Solid Edge part; units mm, degrees
sketch "Sketch1" plane through (0, 0, 0) normal (1, 0, 0) x (0, 1, 0)
  line L0 (0, 50) -> (0, 31)
  line L1 (0, 31) -> (-5, 31)
  line L2 (-5, 31) -> (-5, 26.5)
  line L3 (-5, 26.5) -> (0, 26.5)
  line L4 (0, 26.5) -> (0, 21)
  line L5 (0, 21) -> (4, 21)
  line L6 (4, 21) -> (4, 22.5)
  line L7 (4, 22.5) -> (11, 22.5)
  line L8 (11, 22.5) -> (11, 31)
  line L9 (11, 31) -> (8, 31)
  line L10 (8, 32.5) -> (8, 31)
  line L11 (8, 39) -> (8, 32.5)
  line L12 (8, 39) -> (8, 50)
  line L13 (8, 50) -> (0, 50)
revolve "RevolvedProtrusion1" add sketch "Sketch1" angle 360 about axis through (0, -22.1591, 0) along (0, 1, 0)
sketch "Sketch2" plane through (0, 8, 0) normal (0, 1, 0) x (-1, 0, 0)
  circle A0 centre (-28.2843, -28.2843) radius 4.25
  circle A1 centre (-28.2843, 28.2843) radius 4.25
  circle A2 centre (28.2843, 28.2843) radius 4.25
  circle A3 centre (28.2843, -28.2843) radius 4.25
extrude "Cutout1" cut sketch "Sketch2" against normal blind 16.0733
Check sheet for the modelled part. Datum: model origin and axes. Units: mm. A direction names the side the tool comes from. Coordinates: 2 decimals unless noted, no trailing zeros. Loops run counter-clockwise (first coordinate to the right, second up) from the corner with the lowest first, then second, coordinate; pieces in that order, holes last. Notation, with made-up numbers: (46.5, -35.75) -> (105.5, -35.75) arc R5 ccw to (105.5, -31.75) -> close; hole circle Ø3 at (10, 52). An arc over 180 degrees is marked (long way). Write item = value, one per line. Start each with the question number.
1. Material ranges on line 1 (Z direction, x = -27, y = 5); line 2 (X direction, y = 7.25, z = 0); line 3 (Y direction, x = 33.5, z = 16), recorded low to high.
2. Section check D-D on y = 9.5. Record the cut outline in (x, z), then the cut area to 3 significant figures.
3. Section check B-B on x = 0. Record the cut outline in (y, z), then the cut area to 3 significant figures.
4. Section check A-A on z = 0. Record the cut outline in (x, y).
5. Depth check by flat-ended pin: P1, Ø5, axis at x = 28.28, z = 28.28, coming from the -Y side; P2, Ø16, axis at x = -12, z = 5.5, coming from the -Y side; P3, Ø8, axis at x = -35, y = 0.5, coming from the -Z side; P4, Ø2, axis at y = -3, z = 6.5, coming from the -X side. Enter the tip coordinate at first touch or a pass-through.
6. Tool access check on faces 4 (the flat face through (14, -5, 23)), 5 (the cylindrical face through (-30.736, -2.535, -4.036)), 6 (the flat face through (-22, 8, -23)). Record the directions out of +Z, -Z, +X, -X, +Y, -Y that give a thin tool (end or side, any length) a straight path to the whole face; none if there is none.
7. Section check C-C on y = -2.75. Record the cut outline in (x, z), then the cut area to 3 significant figures.
8. Draft check along Z on faces 1 (the cylindrical face through (-30.736, 9.479, -4.036)), 2 (the flat face through (7, 4, 20)), 3 (the flat face through (-22, 0, -23)). Enter one of: released by +Z, released by -Z, zero draft, split by the parting line, or undercut.
Responses:
q1.line_1 = -42.08 to -32.34, -24.23 to 24.23, 32.34 to 42.08
q1.line_2 = -50 to -22.5, 22.5 to 50
q1.line_3 = 0 to 8
q2.outline = circle Ø62 at (0, 0); hole circle Ø45 at (0, 0)
q2.area = 1,430 mm2
q3.outline = (-5, -31) -> (0, -31) -> (0, -50) -> (8, -50) -> (8, -31) -> (11, -31) -> (11, -22.5) -> (4, -22.5) -> (4, -21) -> (0, -21) -> (0, -26.5) -> (-5, -26.5) -> close; (-5, 26.5) -> (0, 26.5) -> (0, 21) -> (4, 21) -> (4, 22.5) -> (11, 22.5) -> (11, 31) -> (8, 31) -> (8, 50) -> (0, 50) -> (0, 31) -> (-5, 31) -> close
q3.area = 548 mm2
q4.outline = (-50, 0) -> (-31, 0) -> (-31, -5) -> (-26.5, -5) -> (-26.5, 0) -> (-21, 0) -> (-21, 4) -> (-22.5, 4) -> (-22.5, 11) -> (-31, 11) -> (-31, 8) -> (-50, 8) -> close; (21, 0) -> (26.5, 0) -> (26.5, -5) -> (31, -5) -> (31, 0) -> (50, 0) -> (50, 8) -> (31, 8) -> (31, 11) -> (22.5, 11) -> (22.5, 4) -> (21, 4) -> close
q5.P1 = through
q5.P2 = 0
q5.P3 = -39.23
q5.P4 = -30.51
q6.face_4 = +Z, -Z, +X, -X, -Y
q6.face_5 = -Y
q6.face_6 = +Y
q7.outline = circle Ø62 at (0, 0); hole circle Ø53 at (0, 0)
q7.area = 813 mm2
q8.face_1 = split by the parting line
q8.face_2 = undercut
q8.face_3 = zero draft
